Here's how the part is built. I have some questions about the finished solid (model axes, mm). A direction names the side the tool comes from. Give positions to 0.01 mm unless a question says otherwise; leave off trailing zeros. Write each loop counter-clockwise with the first axis right and the second up, starting at its lowest first coordinate (ties: lowest second). Pieces come first, ordered by that corner, then holes. Notation, with made-up numbers: (7, 31.5) -> (62, 31.5) arc R19 cw to (62, 62.5) -> close; hole circle Ø4 at (31.25, -40). An arc over 180 degrees is marked (long way). Return JSON: item names as keys, results as strings.
from build123d import *

# Parameters (mm, degrees)
SKETCH_W        = 27.4
SKETCH_H        = 35
PAD_DEPTH       = 2
SKETCH001_W     = 12
SKETCH001_H     = 14
POCKET_DEPTH    = 2
SKETCH002_W     = 7.7
SKETCH002_H     = 3
PAD001_DEPTH    = 12
FILLET_R        = 3
SKETCH003_W     = 7.7
SKETCH003_H     = 3
PAD002_DEPTH    = 5
FILLET001_R     = 3
SKETCH004_R     = 1.05
POCKET001_DEPTH = 2
SKETCH005_R     = 1.65
POCKET002_DEPTH = 3
FILLET002_R     = 2


with BuildPart() as part:
    # Sketch → Pad (new body)
    with BuildSketch(Plane.XY):
        with Locations((13.7, 17.5)):
            Rectangle(SKETCH_W, SKETCH_H)
    extrude(amount=PAD_DEPTH)

    # Sketch001 (on Face6 of Pad) → Pocket (cut)
    with BuildSketch(Plane.XY.offset(2)):
        with Locations((13.7, 7)):
            Rectangle(SKETCH001_W, SKETCH001_H)
    extrude(amount=-POCKET_DEPTH, mode=Mode.SUBTRACT)

    # Sketch002 (on Face4 of Pocket) → Pad001 (join)
    with BuildSketch(Plane.XY.offset(2)):
        with Locations((3.85, 1.5)):
            Rectangle(SKETCH002_W, SKETCH002_H)
        with Locations((23.55, 1.5)):
            Rectangle(SKETCH002_W, SKETCH002_H)
    extrude(amount=PAD001_DEPTH)

    # Fillet
    fillet_edges = [part.edges().sort_by_distance(p)[0] for p in [
        (3.85, 3, 2),
        (23.55, 3, 2),
    ]]
    fillet(fillet_edges, radius=FILLET_R)

    # Sketch003 (on Face5 of Fillet) → Pad002 (join)
    with BuildSketch(Plane(origin=(0, 0, 0), x_dir=(1, 0, 0), z_dir=(0, 0, -1))):
        with Locations((3.85, -1.5)):
            Rectangle(SKETCH003_W, SKETCH003_H)
        with Locations((23.55, -1.5)):
            Rectangle(SKETCH003_W, SKETCH003_H)
    extrude(amount=PAD002_DEPTH)

    # Fillet001
    fillet001_edges = [part.edges().sort_by_distance(p)[0] for p in [
        (3.85, 3, 0),
        (23.55, 3, 0),
    ]]
    fillet(fillet001_edges, radius=FILLET001_R)

    # Sketch004 (on Face5 of Fillet001) → Pocket001 (cut)
    with BuildSketch(Plane.XY.offset(2)):
        with Locations((3.25, 32.6)):
            Circle(SKETCH004_R)
        with Locations((3.25, 20.1)):
            Circle(SKETCH004_R)
        with Locations((24.15, 32.6)):
            Circle(SKETCH004_R)
        with Locations((24.009843, 20.1)):
            Circle(SKETCH004_R)
    extrude(amount=-POCKET001_DEPTH, mode=Mode.SUBTRACT)

    # Sketch005 (on Face24 of Pocket001) → Pocket002 (cut)
    with BuildSketch(Plane(origin=(0, 3, 0), x_dir=(-1, 0, 0), z_dir=(0, 1, 0))):
        with Locations((-3.8, 9.553689)):
            Circle(SKETCH005_R)
        with Locations((-23.6, 9.553689)):
            Circle(SKETCH005_R)
    extrude(amount=-POCKET002_DEPTH, mode=Mode.SUBTRACT)

    # Fillet002
    fillet002_edges = [part.edges().sort_by_distance(p)[0] for p in [
        (0, 35, 1),
        (27.4, 35, 1),
    ]]
    fillet(fillet002_edges, radius=FILLET002_R)


solid = part.part
1. Suppose I cut it at D-D, the plane y = 11. List the corners of the cut face in (x, z) for me, and give its area (3 significant figures).
Taken from the geometry:
{"outline": "(0, 0) -> (7.7, 0) -> (7.7, 2) -> (0, 2) -> close; (19.7, 0) -> (27.4, 0) -> (27.4, 2) -> (19.7, 2) -> close", "area": "30.8 mm²"}
2. Suppose I cut it at A-A, the plane y = 20.1. List the corners of the cut face in (x, z) for me, and give its area (3 significant figures).
Taken from the geometry:
{"outline": "(0, 0) -> (2.2, 0) -> (2.2, 2) -> (0, 2) -> close; (4.3, 0) -> (22.96, 0) -> (22.96, 2) -> (4.3, 2) -> close; (25.06, 0) -> (27.4, 0) -> (27.4, 2) -> (25.06, 2) -> close", "area": "46.4 mm²"}
3. If I drill on line 1 (Y direction, x = 3.25, z = 1.55); line 2 (Z direction, x = 3.8, y = 2.3); line 3 (X direction, y = 1, z = 9.5), over which ranges is the centre line in solid material (lowest first)? Write a range as [from, to].
Taken from the geometry:
{"line 1": "y = [0, 19.05], [21.15, 31.55], [33.65, 35]", "line 2": "z = [-5, 7.9], [11.2, 14]", "line 3": "x = [0, 2.15], [5.45, 7.7], [19.7, 21.95], [25.25, 27.4]"}
4. Suppose I cut it at C-C, the plane z = -2.5. List the corners of the cut face in (x, y) for me, and give its area (3 significant figures).
Taken from the geometry:
{"outline": "(0, 0) -> (7.7, 0) -> (7.7, 3.04) -> (0, 3.04) -> close; (19.7, 0) -> (27.4, 0) -> (27.4, 3.04) -> (19.7, 3.04) -> close", "area": "46.8 mm²"}
5. Which directions (+Z, -Z, +X, -X, +Y, -Y) give clear straight access to the entire face, cutting with the end or side of a thin tool? Please do faces 5 (the face through (4, 1, -5)), 6 (the face through (14, 21, 2)), 7 (the face through (7.7, 3, 3)).
Taken from the geometry:
{"face 5": "-Z, +X, -X, +Y, -Y", "face 6": "+Z, +X, -X, +Y", "face 7": "+Z, -Z, -Y"}
6. If we mould it in two halves opening along X, with no side actions, what happens to faces 1 (the face through (23.6, 3.9, -0.86)), 2 (the face through (4.01, 1.52, 11.19)), 3 (the face through (26.8, 34.43, 1.01)), 4 (the face through (0, 10.5, 1.7))? For each: released by +X, released by -X, zero draft, split by the parting line, or undercut.
Taken from the geometry:
{"face 1": "zero draft", "face 2": "undercut", "face 3": "released by +X", "face 4": "released by -X"}
7. For pin 1 Ø2.5 at (x, y) = (3.25, 20.1) entering from -Z; pin 2 Ø8.5 at (x, z) = (2, 9) entering from +Y; pin 3 Ø1.3 at (x, y) = (3.25, 32.6) entering from -Z; pin 4 Ø2 at (x, z) = (13.5, 0.5) entering from -Y, each with a flat end and sliding along its axis, tell me the tip position at first contact or that it passes through.
Taken from the geometry:
{"pin 1": "stops at z = 0", "pin 2": "stops at y = 3.01", "pin 3": "passes through", "pin 4": "stops at y = 14"}
8. Suppose I cut it at B-B, the plane x = 3.75. List the corners of the cut face in (y, z) for me.
Taken from the geometry:
{"outline": "(0, -5) -> (3, -5) -> (3, -3) arc R3 cw to (6, 0) -> (19.18, 0) -> (19.18, 2) -> (6, 2) arc R3 cw to (3, 5) -> (3, 7.9) -> (0, 7.9) -> close; (0, 11.2) -> (3, 11.2) -> (3, 14) -> (0, 14) -> close; (21.02, 0) -> (31.68, 0) -> (31.68, 2) -> (21.02, 2) -> close; (33.52, 0) -> (35, 0) -> (35, 2) -> (33.52, 2) -> close"}
